```python
from build123d import *

# Parameters (mm, degrees)
BOSS_EXTRUDE1_DEPTH = 6.35
CAVITY2_START       = -19.049999998
CAVITY2_OUTLINE_W   = 9.525
CAVITY2_OUTLINE_H   = 6.35
CAVITY2_OUTLINE_W_2 = 6.35
CAVITY2_DEPTH       = 6.35
CAVITY2_START_2     = -6.349999998
CAVITY2_2_OUTLINE_W = 6.35
CAVITY2_2_OUTLINE_H = 6.35
CAVITY2_2_DEPTH     = 6.35
CAVITY2_START_3     = 6.350000002
CAVITY2_3_OUTLINE_W = 6.35
CAVITY2_3_OUTLINE_H = 6.35
CAVITY2_3_DEPTH     = 6.35
CAVITY2_START_4     = 19.050000002
CAVITY2_4_OUTLINE_W = 6.35
CAVITY2_4_OUTLINE_H = 6.35
CAVITY2_4_DEPTH     = 6.35
CAVITY2_START_5     = 31.750000002
CAVITY2_5_OUTLINE_W = 6.35
CAVITY2_5_OUTLINE_H = 6.35
CAVITY2_5_DEPTH     = 6.35
CAVITY2_START_6     = 44.450000002
CAVITY2_6_OUTLINE_W = 6.35
CAVITY2_6_OUTLINE_H = 6.35
CAVITY2_6_DEPTH     = 6.35
CAVITY2_START_7     = 57.150000002
CAVITY2_7_OUTLINE_W = 6.35
CAVITY2_7_OUTLINE_H = 6.35
CAVITY2_7_DEPTH     = 6.35
CAVITY2_START_8     = 69.850000002
CAVITY2_8_OUTLINE_W = 6.35
CAVITY2_8_OUTLINE_H = 6.35
CAVITY2_8_DEPTH     = 6.35
CAVITY2_START_9     = 82.550000002
CAVITY2_9_OUTLINE_W = 6.35
CAVITY2_9_OUTLINE_H = 6.35
CAVITY2_9_DEPTH     = 6.35


# Read off the part's stored shape, not the designer's step: Cavity2
with BuildPart() as part:
    # Sketch1 → Boss-Extrude1 (new body)
    with BuildSketch(Plane.XY):
        with BuildLine():
            Line((-19.049999998, -37.547541155), (6.350000002, -37.547541155))
            Line((6.350000002, -37.547541155), (6.350000002, -62.947541155))
            Line((6.350000002, -62.947541155), (69.850000002, -62.947541155))
            ThreePointArc((69.850000002, -62.947541155), (87.810512244, -70.387028913), (95.250000002, -88.347541155))
            Line((95.250000002, -88.347541155), (95.250000002, -139.147541155))
            Line((95.250000002, -139.147541155), (-19.049999998, -139.147541155))
            Line((-19.049999998, -139.147541155), (-19.049999998, -37.547541155))
        make_face()
    extrude(amount=-BOSS_EXTRUDE1_DEPTH)

    # Cavity2 outline → Cavity2 (cut)
    with BuildSketch(Plane.YZ.offset(CAVITY2_START)):
        with Locations((-134.385041155, -3.175)):
            Rectangle(CAVITY2_OUTLINE_W, CAVITY2_OUTLINE_H)
        with Locations((-120.097541155, -3.175)):
            Rectangle(CAVITY2_OUTLINE_W_2, CAVITY2_OUTLINE_H)
        with Locations((-107.397541155, -3.175)):
            Rectangle(CAVITY2_OUTLINE_W_2, CAVITY2_OUTLINE_H)
        with Locations((-94.697541155, -3.175)):
            Rectangle(CAVITY2_OUTLINE_W_2, CAVITY2_OUTLINE_H)
        with Locations((-81.997541155, -3.175)):
            Rectangle(CAVITY2_OUTLINE_W_2, CAVITY2_OUTLINE_H)
        with Locations((-69.297541155, -3.175)):
            Rectangle(CAVITY2_OUTLINE_W_2, CAVITY2_OUTLINE_H)
        with Locations((-56.597541155, -3.175)):
            Rectangle(CAVITY2_OUTLINE_W_2, CAVITY2_OUTLINE_H)
        with Locations((-42.310041155, -3.175)):
            Rectangle(CAVITY2_OUTLINE_W, CAVITY2_OUTLINE_H)
    extrude(amount=CAVITY2_DEPTH, mode=Mode.SUBTRACT)

    # Cavity2 2 outline → Cavity2 2 (cut)
    with BuildSketch(Plane.YZ.offset(CAVITY2_START_2)):
        with Locations((-135.972541155, -3.175)):
            Rectangle(CAVITY2_2_OUTLINE_W, CAVITY2_2_OUTLINE_H)
        with Locations((-40.722541155, -3.175)):
            Rectangle(CAVITY2_2_OUTLINE_W, CAVITY2_2_OUTLINE_H)
    extrude(amount=CAVITY2_2_DEPTH, mode=Mode.SUBTRACT)

    # Cavity2 3 outline → Cavity2 3 (cut)
    with BuildSketch(Plane.YZ.offset(CAVITY2_START_3)):
        with Locations((-135.972541155, -3.175)):
            Rectangle(CAVITY2_3_OUTLINE_W, CAVITY2_3_OUTLINE_H)
    extrude(amount=CAVITY2_3_DEPTH, mode=Mode.SUBTRACT)

    # Cavity2 4 outline → Cavity2 4 (cut)
    with BuildSketch(Plane.YZ.offset(CAVITY2_START_4)):
        with Locations((-135.972541155, -3.175)):
            Rectangle(CAVITY2_4_OUTLINE_W, CAVITY2_4_OUTLINE_H)
    extrude(amount=CAVITY2_4_DEPTH, mode=Mode.SUBTRACT)

    # Cavity2 5 outline → Cavity2 5 (cut)
    with BuildSketch(Plane.YZ.offset(CAVITY2_START_5)):
        with Locations((-135.972541155, -3.175)):
            Rectangle(CAVITY2_5_OUTLINE_W, CAVITY2_5_OUTLINE_H)
    extrude(amount=CAVITY2_5_DEPTH, mode=Mode.SUBTRACT)

    # Cavity2 6 outline → Cavity2 6 (cut)
    with BuildSketch(Plane.YZ.offset(CAVITY2_START_6)):
        with Locations((-135.972541155, -3.175)):
            Rectangle(CAVITY2_6_OUTLINE_W, CAVITY2_6_OUTLINE_H)
    extrude(amount=CAVITY2_6_DEPTH, mode=Mode.SUBTRACT)

    # Cavity2 7 outline → Cavity2 7 (cut)
    with BuildSketch(Plane.YZ.offset(CAVITY2_START_7)):
        with Locations((-135.972541155, -3.175)):
            Rectangle(CAVITY2_7_OUTLINE_W, CAVITY2_7_OUTLINE_H)
    extrude(amount=CAVITY2_7_DEPTH, mode=Mode.SUBTRACT)

    # Cavity2 8 outline → Cavity2 8 (cut)
    with BuildSketch(Plane.YZ.offset(CAVITY2_START_8)):
        with Locations((-135.972541155, -3.175)):
            Rectangle(CAVITY2_8_OUTLINE_W, CAVITY2_8_OUTLINE_H)
    extrude(amount=CAVITY2_8_DEPTH, mode=Mode.SUBTRACT)

    # Cavity2 9 outline → Cavity2 9 (cut)
    with BuildSketch(Plane.YZ.offset(CAVITY2_START_9)):
        with Locations((-135.972541155, -3.175)):
            Rectangle(CAVITY2_9_OUTLINE_W, CAVITY2_9_OUTLINE_H)
    extrude(amount=CAVITY2_9_DEPTH, mode=Mode.SUBTRACT)


solid = part.part
```
Model file for the job. Use its own axes, mm. A direction names the side the tool comes from. Coordinates: 2 decimals unless noted, no trailing zeros. Write each loop counter-clockwise with the first axis right and the second up, starting at its lowest first coordinate (ties: lowest second). Pieces come first, ordered by that corner, then holes. Notation, with made-up numbers: (28, -18) - (62, -18) arc R16 cw to (62, -12) - close; hole circle Ø1 at (-12, 79). An arc over 180 degrees is marked (long way). Use a Markdown table: item, result. Add a question column.
Item 1: Band-saw the part on A-A, the plane x = 28.5. Write the cut outline in (y, z).
Item 2: Drill centre lines: line 1 along X through (y, z) = (-106, -5.5); line 2 along X through (y, z) = (-54, -3.5); line 3 along Y through (x, z) = (42, -0.5). Where is each one in solid material? Low to high.
Item 3: Band-saw the part on B-B, the plane y = -68. Write the cut outline in (x, z), and give its area (3 significant figures).
Item 4: 3-axis set-ups, long thin cutter, end or side, ignore diameter. For faces 1 (the face through (-12.7, -120, -3)), 2 (the face through (86, -132.798, -3)), 3 (the face through (0, -41, -3)): which of +Z, -Z, +X, -X, +Y, -Y reach the whole face in a straight line?
Item 5: Drop flat-ended pins along their axis: pin 1 (3 mm diameter, centred on x = 59, z = -3.5, fed in from -Y); pin 2 (1.9 mm diameter, centred on x = -16, z = -1.5, fed in from +Y). Give the stop position or say it passes through.
Item 6: Two-plate mould, pull along X, no slides. Class faces 4 (the face through (6.35, -136, -3)), 5 (the face through (38, -62.948, -3)), 6 (the face through (-12.7, -57, -3)): pulls with the +X half, pulls with the -X half, needs draft (parallel to the pull), parting line crosses it, or undercut.
A:
| question | item | result |
|---|---|---|
| 1 | outline | (-139.15, -6.35) - (-62.95, -6.35) - (-62.95, 0) - (-139.15, 0) - close |
| 2 | line 1 | x = -12.7 to 95.25 |
| 2 | line 2 | x = -12.7 to 6.35 |
| 2 | line 3 | y = -139.15 to -62.95 |
| 3 | outline | (-12.7, -6.35) - (85.05, -6.35) - (85.05, 0) - (-12.7, 0) - close |
| 3 | area | 621 mm² |
| 4 | face 1 | +Z, -Z, -X |
| 4 | face 2 | +Z, -Z, -Y |
| 4 | face 3 | +Z, -Z, +Y |
| 5 | pin 1 | stops at y = -132.8 |
| 5 | pin 2 | stops at y = -47.07 |
| 6 | face 4 | undercut |
| 6 | face 5 | needs draft |
| 6 | face 6 | pulls with the -X half |
